Design review of the part built by this model. Coordinates are the model's own, in mm. Face numbers are marked on the shaded views. Coordinates: 2 decimals unless noted, no trailing zeros. Order: outer loops, then holes, each group sorted by start corner. A loop starts at its lowest first (then second) coordinate and runs counter-clockwise, first axis right, second up. Notation, with made-up numbers: (27.5, 84.25) -> (53.5, 84.25) arc R30 cw to (53.5, 109.25) -> close; hole circle Ø8 at (-37, -12.5). An arc over 180 degrees is marked (long way). Use a Markdown table: item, result. Add a question column.
Q1. Insertion check: pin 1 (6 mm diameter, centred on y = 167.5, z = 97, fed in from +X); pin 2 (6 mm diameter, centred on x = -116, y = 118.5, fed in from +Z); pin 3 (3 mm diameter, centred on x = -140, z = 257, fed in from -Y) (3 decimals). Each pin has a flat end and moves straight along its axis. Give the tip position at first contact, or say it passes through.
Q2. Add section B-B (z = 0). State the section outline as (x, y) points (1 decimal), then the cut area to 3 significant figures.
Q3. The part is to be moulded in two halves that separate along Z. For the marked faces 1, 2, 3 and 4, say which applies: pulls with the +Z half, pulls with the -Z half, needs draft (parallel to the pull), parting line crosses it, or undercut.
Q4. Add section C-C (y = 92). State the section outline as (x, z) points (1 decimal).
Q5. Add section A-A (x = 0). State the section outline as (y, z) points (1 decimal), then the cut area to 3 significant figures.
Q6. Wall thickness on probe 1 along Z at (x, y) = (0, 140); probe 2 along Z at (x, y) = (0, 40.8); probe 3 along Y at (x, z) = (154, -280) (3 decimals): over which ranges is each line inside the solid? List them lowest first.
from build123d import *

# Parameters (mm, degrees)
F0_R     = 380.9365
F0_R_2   = 236.5375
F1_DEPTH = 304.8


with BuildPart() as f1:
    # F0 (on Front) → F1 (new body)
    with BuildSketch(Plane.XZ):
        Circle(F0_R)
        Circle(F0_R_2, mode=Mode.SUBTRACT)
    extrude(amount=-F1_DEPTH)

    # F2 (on Right) → F3 (revolve, cut)
    with BuildSketch(Plane.YZ):
        Polygon((-0.674657, 0), (0, 0), (9.525, 0), (9.525, 323.444068), (0, 325.9074), (-38.13795, 325.9074), align=None)
    revolve(axis=Axis((0, -111.905819, 0), (0, -1, 0)), mode=Mode.SUBTRACT)

    # F4 (on Right) → F5 (revolve, cut)
    with BuildSketch(Plane.YZ):
        Polygon((39.294728, 254.3556), (9.525, 266.9921), (-83.954796, 266.9921), (-48.076838, 187.997639), (83.789648, 229.984577), (72.7964, 240.977825), (52.705, 252.5776), (45.438306, 252.5776), (41.2496, 254.3556), align=None)
    revolve(axis=Axis((0, 0, 0), (0, -1, 0)), mode=Mode.SUBTRACT)


solid = f1.part
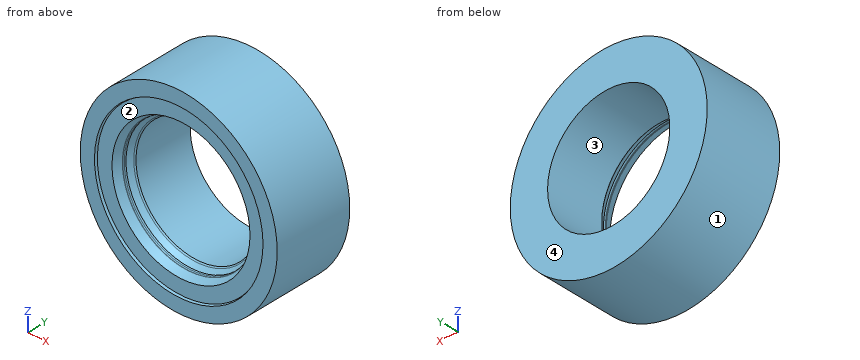
Established:
| question | item | result |
|---|---|---|
| 1 | pin 1 | x = 369.16 |
| 1 | pin 2 | z = 363.79 |
| 1 | pin 3 | y = 9.525 |
| 2 | outline | (-380.9, 0) -> (-325.9, 0) -> (-323.4, 9.5) -> (-267, 9.5) -> (-254.4, 39.3) -> (-254.4, 41.2) -> (-252.6, 45.4) -> (-252.6, 52.7) -> (-241, 72.8) -> (-236.5, 77.2) -> (-236.5, 304.8) -> (-380.9, 304.8) -> close; (236.5, 77.2) -> (241, 72.8) -> (252.6, 52.7) -> (252.6, 45.4) -> (254.4, 41.2) -> (254.4, 39.3) -> (267, 9.5) -> (323.4, 9.5) -> (325.9, 0) -> (380.9, 0) -> (380.9, 304.8) -> (236.5, 304.8) -> close |
| 2 | area | 84,000 mm^2 |
| 3 | face 1 | parting line crosses it |
| 3 | face 2 | undercut |
| 3 | face 3 | undercut |
| 3 | face 4 | needs draft |
| 4 | outline | circle Ø761.9 at (0, 0); hole circle Ø473.1 at (0, 0) |
| 5 | outline | (0, -380.9) -> (304.8, -380.9) -> (304.8, -236.5) -> (77.2, -236.5) -> (72.8, -241) -> (52.7, -252.6) -> (45.4, -252.6) -> (41.2, -254.4) -> (39.3, -254.4) -> (9.5, -267) -> (9.5, -323.4) -> (0, -325.9) -> close; (0, 325.9) -> (9.5, 323.4) -> (9.5, 267) -> (39.3, 254.4) -> (41.2, 254.4) -> (45.4, 252.6) -> (52.7, 252.6) -> (72.8, 241) -> (77.2, 236.5) -> (304.8, 236.5) -> (304.8, 380.9) -> (0, 380.9) -> close |
| 5 | area | 84,000 mm^2 |
| 6 | probe 1 | -380.94 to -236.54, 236.54 to 380.94 |
| 6 | probe 2 | -380.94 to -254.36, 254.36 to 380.94 |
| 6 | probe 3 | 9.525 to 304.8 |
